The model under review builds one solid part; all positions refer to its coordinate system, in mm. Face numbers are marked on the shaded views. A direction names the side the tool comes from. Give positions to 0.01 mm unless a question says otherwise; leave off trailing zeros. Loops run counter-clockwise (first coordinate to the right, second up) from the corner with the lowest first, then second, coordinate; pieces in that order, holes last. Notation, with made-up numbers: M -5.75,18 L 48.25,18 A23 ccw 48.25,42 Z; hole C 18,-28.5 d5. An arc over 180 degrees is marked long. Put each result on its own line as item: value. Start each with the question number.
```python
from build123d import *

# Parameters (mm, degrees)
SKETCH4_R               = 1.2500000000000113
SKETCH4_R_2             = 1.2499999999999978
BOSS_EXTRUDE4_DEPTH     = 2
SKETCH4_5_R             = 1.7500000000000104
SKETCH4_5_R_2           = 1.749999999999997
BOSS_EXTRUDE5_DEPTH     = 9
SKETCH4_6_R             = 1.749999999999997
SKETCH4_6_R_2           = 1.2499999999999978
SKETCH4_6_R_3           = 1.7500000000000104
SKETCH4_6_R_4           = 1.2500000000000113
BOSS_EXTRUDE6_DEPTH     = 3
CUT_EXTRUDE1_DEPTH      = 158.79099158717955
CUT_EXTRUDE1_DEPTH_BACK = 158.79099158717955
FILLET1_R               = 1
FILLET2_R               = 0.25
CUT_EXTRUDE2_DEPTH      = 158.79099158717955
CUT_EXTRUDE2_DEPTH_BACK = 158.79099158717955
CHAMFER1_SIZE           = 0.5


with BuildPart() as part:
    # Sketch4 → Boss-Extrude4 (new body)
    with BuildSketch(Plane.XY):
        with BuildLine():
            add(Edge.make_bspline(
                [(-121.0977219670568, -59.96744638283075), (-120.94298009720131, -59.87814106550356), (-120.8476486211035, -59.71305439455445), (-120.8476486210958, -59.53439134300407)],
                knots=[3, 3, 3, 3, 4, 4, 4, 4], degree=3))
            Line((-120.8476486210958, -59.53439134300407), (-120.8476486189429, -11.586453102615721))
            Line((-120.8476486189429, -11.58645310261572), (-120.8476486189429, -8.0865191630969))
            Line((-120.8476486189429, -8.0865191630969), (-140.5664979509455, -8.083912687906277))
            Line((-140.5664979509455, -8.083912687906277), (-140.5664979509455, -11.58397880929067))
            Line((-140.5664979509455, -11.58397880929067), (-140.5664979535839, -70.33749706476789))
            add(Edge.make_bspline(
                [(-140.5664979535839, -70.33749706476789), (-140.5664979536002, -70.72235960570497), (-140.1499046258814, -70.96292691883274), (-139.8165712997942, -70.7705521046382)],
                knots=[1, 1, 1, 1, 2, 2, 2, 2], degree=3))
            Line((-139.8165712997942, -70.7705521046382), (-121.0977219670568, -59.96744638283075))
        make_face()
        with Locations((-137.92794657478115, -67.08936245467149)):
            Circle(SKETCH4_R, mode=Mode.SUBTRACT)
        with Locations((-123.49593879557014, -58.568434854590414)):
            Circle(SKETCH4_R_2, mode=Mode.SUBTRACT)
    extrude(amount=-BOSS_EXTRUDE4_DEPTH)

    # Sketch4<5> → Boss-Extrude5 (add)
    # profile 1 of 2: a face of its own
    with BuildSketch(Plane.XY):
        Polygon((-140.56649795336358, -65.4304148764118), (-123.8285782795111, -55.7705521046382), (-140.56649795292978, -55.7705521046382), align=None)
    # profile 2 of 2: a face of its own
    with BuildSketch(Plane.XY):
        with BuildLine():
            add(Edge.make_bspline(
                [(-121.0977219670568, -59.96744638283075), (-120.94298009720131, -59.87814106550356), (-120.8476486211035, -59.71305439455445), (-120.8476486210958, -59.53439134300407)],
                knots=[3, 3, 3, 3, 4, 4, 4, 4], degree=3))
            Line((-120.8476486210958, -59.53439134300407), (-120.8476486209268, -55.7705521046382))
            Line((-120.84764862092679, -55.7705521046382), (-123.8285782795111, -55.7705521046382))
            Line((-123.8285782795111, -55.7705521046382), (-140.56649795336358, -65.4304148764118))
            Line((-140.56649795336355, -65.4304148764118), (-140.5664979535839, -70.33749706476789))
            add(Edge.make_bspline(
                [(-140.5664979535839, -70.33749706476789), (-140.5664979536002, -70.72235960570497), (-140.1499046258814, -70.96292691883274), (-139.8165712997942, -70.7705521046382)],
                knots=[1, 1, 1, 1, 2, 2, 2, 2], degree=3))
            Line((-139.8165712997942, -70.7705521046382), (-121.0977219670568, -59.96744638283075))
        make_face()
        with Locations((-137.92794657478115, -67.08936245467149)):
            Circle(SKETCH4_5_R, mode=Mode.SUBTRACT)
        with Locations((-123.49593879557014, -58.568434854590414)):
            Circle(SKETCH4_5_R_2, mode=Mode.SUBTRACT)
    extrude(amount=BOSS_EXTRUDE5_DEPTH)

    # Sketch4<6> → Boss-Extrude6 (add)
    # profile 1 of 2: a face of its own
    with BuildSketch(Plane.XY):
        with Locations((-123.49593879557014, -58.568434854590414)):
            Circle(SKETCH4_6_R)
        with Locations((-123.49593879557014, -58.568434854590414)):
            Circle(SKETCH4_6_R_2, mode=Mode.SUBTRACT)
    # profile 2 of 2: a face of its own
    with BuildSketch(Plane.XY):
        with Locations((-137.92794657478115, -67.08936245467149)):
            Circle(SKETCH4_6_R_3)
        with Locations((-137.92794657478115, -67.08936245467149)):
            Circle(SKETCH4_6_R_4, mode=Mode.SUBTRACT)
    extrude(amount=BOSS_EXTRUDE6_DEPTH)

    # Sketch8 → Cut-Extrude1 (cut, two sides: drawn at the far end of the back side and taken through both)
    with BuildSketch(Plane(origin=(0, 0, -2), x_dir=(-1, 0, 0), z_dir=(0, 0, -1)).offset(-CUT_EXTRUDE1_DEPTH_BACK)):
        with BuildLine():
            Line((139.5664979509455, -49.27055210463822), (143.2884320777397, -49.27055210463822))
            Line((143.2884320777397, -49.27055210463822), (143.2884320777397, -52.270552104638206))
            Line((143.2884320777397, -52.270552104638206), (139.5664979509455, -52.270552104638206))
            ThreePointArc((139.5664979509455, -52.270552104638206), (138.0664979509455, -50.77055210463821), (139.5664979509455, -49.27055210463822))
        make_face()
    extrude(amount=CUT_EXTRUDE1_DEPTH + CUT_EXTRUDE1_DEPTH_BACK, mode=Mode.SUBTRACT)

    # Fillet1
    fillet1_edges = [part.edges().sort_by_distance(p)[0] for p in [
        (-140.06649795193763, -52.270552104638206, 0),
        (-140.06649795227284, -52.270552104638206, -2),
        (-140.06649795193763, -49.27055210463822, 0),
        (-140.06649795227284, -49.27055210463822, -2),
        (-138.0664979509455, -50.77055210463821, 0),
        (-138.0664979509455, -50.77055210463821, -2),
    ]]
    fillet(fillet1_edges, radius=FILLET1_R - 0.0001)  # a hair under: the kernel refuses the full size

    # Fillet2
    fillet2_edges = [part.edges().sort_by_distance(p)[0] for p in [
        (-140.56649795176924, -29.927315456964447, 0),
        (-140.31653462082718, -70.7704885946968, -2),
        (-130.4571466334255, -65.36899924373448, -2),
        (-120.91465709288339, -59.78442801325112, -2),
        (-120.84764862001936, -35.56042222280989, -2),
        (-130.7070732849442, -8.08521592550159, -2),
        (-124.74593879557014, -58.568434854590414, -2),
        (-139.17794657478115, -67.08936245467149, -2),
        (-140.56649795176924, -29.927315456964447, -2),
        (-140.56649795287362, -54.5205021046382, 0),
        (-140.5664979532007, -61.80397458470304, -2),
        (-140.56649795281749, -52.56341603412977, -1.707136070508429),
        (-140.56649795281749, -52.56341603412977, -0.29286392949157103),
        (-140.56649795259295, -48.97768817514665, -1.707136070508429),
        (-140.56649795259295, -48.97768817514665, -0.2928639294915709),
    ]]
    fillet(fillet2_edges, radius=FILLET2_R)

    # Sketch9 → Cut-Extrude2 (cut, two sides: drawn at the far end of the back side and taken through both)
    with BuildSketch(Plane(origin=(0, 0, -2), x_dir=(-1, 0, 0), z_dir=(0, 0, -1)).offset(-CUT_EXTRUDE2_DEPTH_BACK)):
        Polygon((125.95707332644032, -20.085843894406473), (135.45707324344806, -20.084588166261394), (135.45707324344806, -46.08458816626139), (125.95707332644032, -46.08458816626139), align=None)
    extrude(amount=CUT_EXTRUDE2_DEPTH + CUT_EXTRUDE2_DEPTH_BACK, mode=Mode.SUBTRACT)

    # Chamfer1
    chamfer1_edges = [part.edges().sort_by_distance(p)[0] for p in [
        (-125.95707332644032, -33.08521603033393, -2),
        (-130.7070732849442, -20.08521603033393, -2),
        (-135.45707324344806, -33.08458816626139, -2),
        (-130.7070732849442, -46.08458816626139, -2),
    ]]
    chamfer(chamfer1_edges, length=CHAMFER1_SIZE)


solid = part.part
```
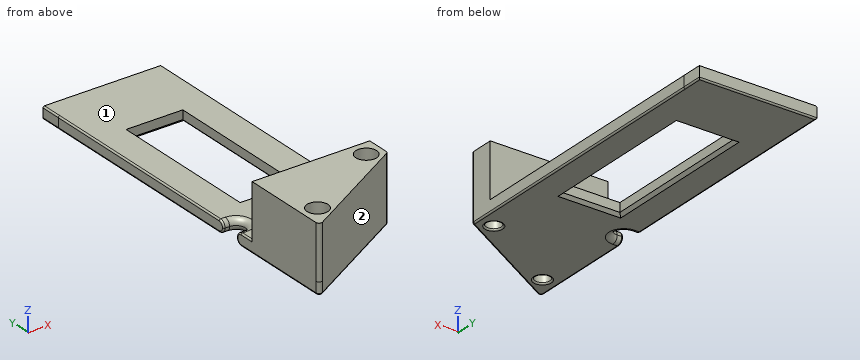
Item 1: To check wall thickness, follow L1, parallel to Y at x = -122.5, z = 6.75; L2, parallel to Y at x = -125, z = 3.75; L3, parallel to Z at x = -136.5, y = -15. State the ranges of each line that lie inside material, in increasing order. Write a range as [from, to].
Item 2: Consider section C-C, the plane z = 5. Give the number of separate pieces and of enclosed holes in the cut face, plus the area to 3 significant figures.
Item 3: Clearance check with flat-ended pins moving along their axes: pin 1 Ø1.8 at (x, y) = (-138.5, -67.5) entering from +Z; pin 2 Ø6 at (x, z) = (-129.5, 4.5) entering from +Y; pin 3 Ø1 at (x, z) = (-135, 2) entering from -Y. State where each tip first meets the part, or that it passes through.
Item 4: Consider section A-A, the plane y = -40.5. Write out the cut boundary in (x, z).
Item 5: Tool access review of the marked faces 1 and 2: name each direction out of +Z, -Z, +X, -X, +Y, -Y from which nothing blocks a thin tool from reaching the whole face with its end or side.
Item 6: Consider section B-B, the plane y = -17. Write out the cut boundary in (x, z), plus the area to 3 significant figures.
Report:
1. L1: [-60.78, -60.01], [-57.13, -55.77]
1. L2: [-62.22, -59.46], [-57.67, -55.77]
1. L3: [-2, 0]
2. separate pieces: 1
2. enclosed holes: 2
2. area: 173 mm²
3. pin 1: z = 3
3. pin 2: y = -55.77
3. pin 3: y = -68.28
4. outline: M -140.57,-1.75 A0.25 ccw -140.32,-2 L -135.96,-2 L -135.46,-1.5 L -135.46,0 L -140.32,0 A0.25 ccw -140.57,-0.25 Z; M -125.96,-1.5 L -125.46,-2 L -121.1,-2 A0.25 ccw -120.85,-1.75 L -120.85,0 L -125.96,0 Z
5. face 1: +Z, +X, -X, +Y
5. face 2: +Z, -Z, +X, -Y
6. outline: M -140.57,-1.75 A0.25 ccw -140.32,-2 L -121.1,-2 A0.25 ccw -120.85,-1.75 L -120.85,0 L -140.32,0 A0.25 ccw -140.57,-0.25 Z
6. area: 39.4 mm²
